Check sheet for the modelled part. Datum: model origin and axes. Units: mm. Face numbers are marked on the shaded views. A direction names the side the tool comes from. Round coordinates to 2 decimals unless told otherwise and drop trailing zeros. Loops run counter-clockwise (first coordinate to the right, second up) from the corner with the lowest first, then second, coordinate; pieces in that order, holes last. Notation, with made-up numbers: (73.25, -20.75) - (131.25, -20.75) arc R25 cw to (131.25, 18.25) - close; hole circle Ø6 at (74.5, 52.25). An arc over 180 degrees is marked (long way). Answer in a Markdown table with one row per item. Add a question column.
(1) Cross-section at C-C on y = 9. Enter the section's corners in (x, z), then the cut area to 3 significant figures.
(2) Cross-section at B-B on x = -6.5. Enter the section's corners in (y, z), then the cut area to 3 significant figures.
(3) Cross-section at D-D on y = 17.5. Enter the section's corners in (x, z), then the cut area to 3 significant figures.
(4) Cross-section at A-A on z = 39. Enter the section's corners in (x, y).
(5) Access from +Z, -Z, +X, -X, +Y, -Y to the whole of each face (thin tool, end or side, straight path). Record for the marked faces 1 and 2.
(6) Thickness scan on line 1 along X through (y, z) = (4.5, 25.5); line 2 along X through (y, z) = (6.25, 35.5); line 3 along Y through (x, z) = (-15.25, 22.5). Record the ranges inside material, lowest first.
(7) Gauge pin test, flat ends, axial feed: pin 1 (1.5 mm diameter, centred on x = -1, z = 20.5, fed in from +Y); pin 2 (3 mm diameter, centred on x = -11.5, z = 59.5, fed in from +Y); pin 3 (12 mm diameter, centred on x = -13.5, y = 15, fed in from +Z). Record the tip position at first contact, or that the pin passes through.
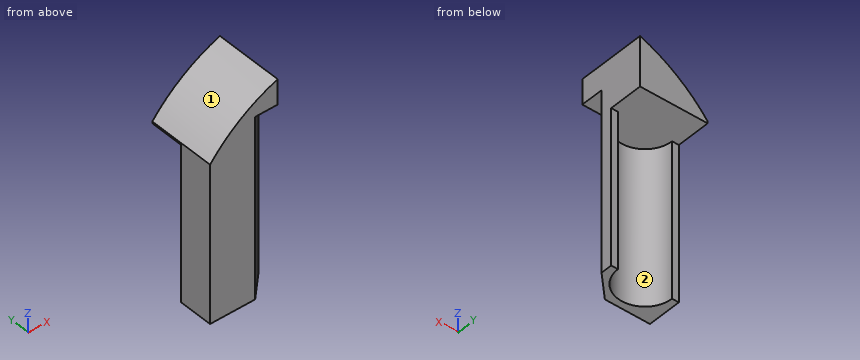
from build123d import *

# Parameters (mm, degrees)
SKETCH2_W           = 30
SKETCH2_H           = 30
BOSS_EXTRUDE1_DEPTH = 100
CUT_EXTRUDE1_START  = -30
CUT_EXTRUDE1_DEPTH  = 30
CUT_EXTRUDE2_DEPTH  = 69
CUT_EXTRUDE3_DEPTH  = 80


# Read off the part's stored shape, not the designer's step: Cut-Extrude1
with BuildPart() as part:
    # Sketch2 → Boss-Extrude1 (new body)
    with BuildSketch(Plane.XY):
        with Locations((-15, 15)):
            Rectangle(SKETCH2_W, SKETCH2_H)
    extrude(amount=BOSS_EXTRUDE1_DEPTH)

    # Cut-Extrude1 outline → Cut-Extrude1 (cut)
    with BuildSketch(Plane.XZ.offset(CUT_EXTRUDE1_START)):
        with BuildLine():
            ThreePointArc((-30, 69.824648593), (-16.445900415, 82.511221459), (0, 91.124879576))
            Line((0, 91.124879576), (0, 100))
            Line((0, 100), (-30, 100))
            Line((-30, 100), (-30, 69.824648593))
        make_face()
    extrude(amount=CUT_EXTRUDE1_DEPTH, mode=Mode.SUBTRACT)

    # Sketch4 → Cut-Extrude2 (cut)
    with BuildSketch(Plane(origin=(0, 0, 0), x_dir=(-1, 0, 0), z_dir=(0, 0, -1))):
        with BuildLine():
            Line((3, 15), (0, 15))
            Line((0, 15), (0, 30))
            Line((0, 30), (30, 30))
            Line((30, 30), (30, 15))
            Line((30, 15), (27, 15))
            ThreePointArc((27, 15), (15, 3), (3, 15))
        make_face()
    extrude(amount=-CUT_EXTRUDE2_DEPTH, mode=Mode.SUBTRACT)

    # Sketch5 → Cut-Extrude3 (cut)
    with BuildSketch(Plane(origin=(0, 0, 0), x_dir=(-1, 0, 0), z_dir=(0, 0, -1))):
        Polygon((0, 0), (0, 10), (10, 0), align=None)
    extrude(amount=-CUT_EXTRUDE3_DEPTH, mode=Mode.SUBTRACT)


solid = part.part
Answers:
| question | item | result |
|---|---|---|
| 1 | outline | (-30, 0) - (-25.39, 0) - (-25.39, 69) - (-4.61, 69) - (-4.61, 0) - (-1, 0) - (-1, 80) - (0, 80) - (0, 91.12) arc R69 ccw to (-30, 69.82) - close |
| 1 | area | 962 mm^2 |
| 2 | outline | (0, 80) - (3.5, 80) - (3.5, 0) - (6.53, 0) - (6.53, 69) - (30, 69) - (30, 88.39) - (0, 88.39) - close |
| 2 | area | 752 mm^2 |
| 3 | outline | (-30, 69) - (0, 69) - (0, 91.12) arc R69 ccw to (-30, 69.82) - close |
| 3 | area | 406 mm^2 |
| 4 | outline | (-30, 0) - (-10, 0) - (0, 10) - (0, 15) - (-3, 15) arc R12 cw to (-27, 15) - (-30, 15) - close |
| 5 | face 1 | +Z, -X, +Y, -Y |
| 5 | face 2 | -Z, +Y |
| 6 | line 1 | x = -30 to -20.81, -9.19 to -5.5 |
| 6 | line 2 | x = -30 to -23.21, -6.79 to -3.75 |
| 6 | line 3 | y = 0 to 3 |
| 7 | pin 1 | stops at y = 15 |
| 7 | pin 2 | stops at y = 4.09 |
| 7 | pin 3 | stops at z = 87.89 |
